Print and shaded views of the part. All mm, measured from the part's lowest x, y and z. A direction names the side the tool comes from. Give positions to 0.01 mm unless a question says otherwise; leave off trailing zeros. Write each loop counter-clockwise with the first axis right and the second up, starting at its lowest first coordinate (ties: lowest second). Pieces come first, ordered by that corner, then holes. Notation, with made-up numbers: (25, -36) -> (46, -36) arc R21 cw to (46, -22) -> close; hole circle Ø2 at (-30, 42.25). An arc over 180 degrees is marked (long way). Put each result on its own line as item: value.
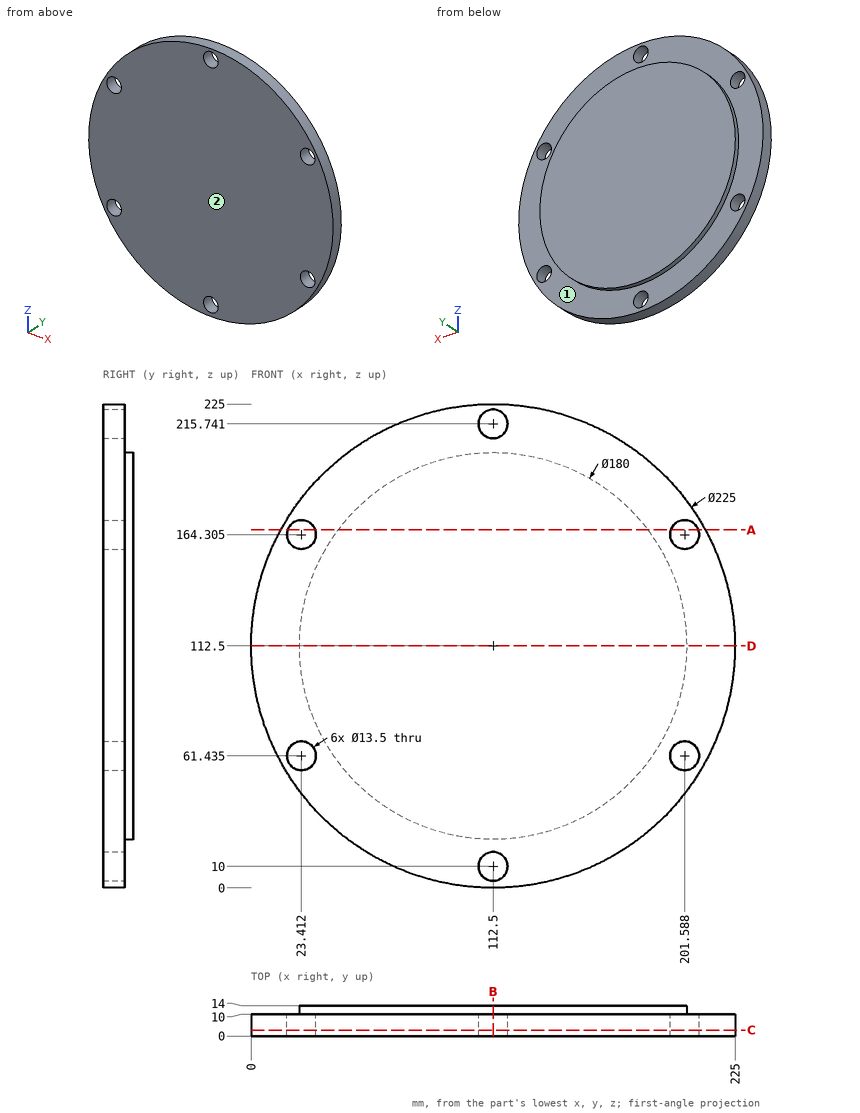
1) Slice it at D-D (z = 112.5). Write the cut outline in (x, y).
Filled sheet:
outline: (0, 0) -> (225, 0) -> (225, 10) -> (202.5, 10) -> (202.5, 14) -> (22.5, 14) -> (22.5, 10) -> (0, 10) -> close
2) Slice it at C-C (y = 2.75). Give the number of separate pieces and of enclosed holes in the cut face, plus the area to 3 significant figures.
Filled sheet:
separate pieces: 1
enclosed holes: 6
area: 38,900 mm2
3) Wall check: L1, parallel to Z at x = 114, y = 6.75; L2, parallel to Y at x = 22.5, z = 108; L3, parallel to X at y = 9.5, z = 161 (1 decimal). Give the ranges that are in metal, low to high.
Filled sheet:
L1: 0.01 to 3.42, 16.58 to 209.16, 222.32 to 224.99
L2: 0 to 10
L3: 11 to 17.5, 29.3 to 195.7, 207.5 to 214
4) Slice it at B-B (x = 112.5). Write the cut outline in (y, z).
Filled sheet:
outline: (0, 0) -> (10, 0) -> (10, 3.25) -> (0, 3.25) -> close; (0, 16.75) -> (10, 16.75) -> (10, 22.5) -> (14, 22.5) -> (14, 202.5) -> (10, 202.5) -> (10, 208.99) -> (0, 208.99) -> close; (0, 222.49) -> (10, 222.49) -> (10, 225) -> (0, 225) -> close
5) Pin check, flat tips, straight feed: pin 1 (1.5 mm diameter, centred on x = 127.5, y = 3.5, fed in from -Z); pin 2 (15.5 mm diameter, centred on x = 201.59, z = 164.31, fed in from -Y); pin 3 (5 mm diameter, centred on x = 163, y = 11.5, fed in from -Z); pin 4 (21.5 mm diameter, centred on x = 112.5, z = 10, fed in from +Y). Stop position of each tip, or through.
Filled sheet:
pin 1: z = 0.91
pin 2: y = 0
pin 3: z = 10.99
pin 4: y = 10
6) Tool access for the marked faces 1 and 2: list every direction of +Z, -Z, +X, -X, +Y, -Y with a clear straight run to the whole face (end or side of a thin tool).
Filled sheet:
face 1: +Y
face 2: +Z, -Z, +X, -X, -Y
7) Slice it at A-A (z = 166.5). Write the cut outline in (x, y) (1 decimal), plus the area to 3 significant figures.
Filled sheet:
outline: (13.8, 0) -> (17, 0) -> (17, 10) -> (13.8, 10) -> close; (29.8, 0) -> (195.2, 0) -> (195.2, 10) -> (184.5, 10) -> (184.5, 14) -> (40.5, 14) -> (40.5, 10) -> (29.8, 10) -> close; (208, 0) -> (211.2, 0) -> (211.2, 10) -> (208, 10) -> close
area: 2,290 mm2
